```python
from build123d import *

# Parameters (mm, degrees)
SKETCH1_W           = 45.21
SKETCH1_H           = 20.09
SKETCH1_R           = 1.13
BOSS_EXTRUDE1_DEPTH = 1.2
SKETCH2_W           = 6
SKETCH2_H           = 16
BOSS_EXTRUDE3_DEPTH = 9
CUT_EXTRUDE1_REACH  = 32.67
SKETCH5_W           = 8
SKETCH5_H           = 9
BOSS_EXTRUDE5_DEPTH = 4


with BuildPart() as part:
    # Sketch1 → Boss-Extrude1 (new body)
    with BuildSketch(Plane(origin=(0, 0, 0), x_dir=(1, 0, 0), z_dir=(0, 1, 0))):
        Rectangle(SKETCH1_W, SKETCH1_H)
        with Locations(Location((11.835, 7.785, 0), (0, 0, 270))):
            Circle(SKETCH1_R, mode=Mode.SUBTRACT)
        with Locations(Location((-20.675, -7.635, 0), (0, 0, 270))):
            Circle(SKETCH1_R, mode=Mode.SUBTRACT)
    extrude(amount=BOSS_EXTRUDE1_DEPTH)

    # Sketch2 → Boss-Extrude3 (add)
    with BuildSketch(Plane(origin=(0, 1.2, 0), x_dir=(1, 0, 0), z_dir=(0, 1, 0))):
        with Locations((18.605, 0)):
            Rectangle(SKETCH2_W, SKETCH2_H)
    extrude(amount=BOSS_EXTRUDE3_DEPTH)

    # Sketch4 → Cut-Extrude1 (cut, up to next)
    with BuildSketch(Plane.XY.offset(8), mode=Mode.PRIVATE) as cut_extrude1_sk1:
        Polygon((15.605, 5.7), (16.788227765, 10.2), (15.605, 10.2), align=None)
    cut_extrude1_tool1 = extrude(cut_extrude1_sk1.sketch, amount=-CUT_EXTRUDE1_REACH, mode=Mode.PRIVATE) & part.part
    # Sketch4 → Cut-Extrude1 (cut, up to next)
    with BuildSketch(Plane.XY.offset(8), mode=Mode.PRIVATE) as cut_extrude1_sk2:
        Polygon((20.317369028, 10.2), (21.605, 5.7), (21.605, 10.2), align=None)
    cut_extrude1_tool2 = extrude(cut_extrude1_sk2.sketch, amount=-CUT_EXTRUDE1_REACH, mode=Mode.PRIVATE) & part.part
    add(cut_extrude1_tool1.solids().sort_by_distance((15.999409, 8.7, 8))[0], mode=Mode.SUBTRACT)
    add(cut_extrude1_tool2.solids().sort_by_distance((21.17579, 8.7, 8))[0], mode=Mode.SUBTRACT)

    # Sketch5 → Boss-Extrude5 (add)
    with BuildSketch(Plane(origin=(0, 1.2, 0), x_dir=(1, 0, 0), z_dir=(0, 1, 0))):
        with Locations((-13.605, -5.545)):
            Rectangle(SKETCH5_W, SKETCH5_H)
    extrude(amount=BOSS_EXTRUDE5_DEPTH)


solid = part.part
```
Verification items for the finished model (mm, model axes). A direction names the side the tool comes from. Round coordinates to 2 decimals unless told otherwise and drop trailing zeros. Order: outer loops, then holes, each group sorted by start corner. A loop starts at its lowest first (then second) coordinate and runs counter-clockwise, first axis right, second up. Notation, with made-up numbers: (25, 74.5) -> (77, 74.5) arc R12 ccw to (77, 80.5) -> close; hole circle Ø3 at (43, 12.25). An arc over 180 degrees is marked (long way). Put each result on its own line as item: value. Start each with the question number.
(1) Section check B-B (z = 5.5). Enter the section's corners in (x, y) (3 decimals).
(2) Material ranges on line 1 along X through (y, z) = (5, 5.75) (3 decimals); line 2 along Z through (x, y) = (-14, 5) (3 decimals); line 3 along Y through (x, z) = (13, 0.75), recorded low to high.
(3) Section check D-D (z = -5.25). Enter the section's corners in (x, y) (3 decimals), then the cut area to 3 significant figures.
(4) Section check A-A (y = 4). Enter the section's corners in (x, z) (3 decimals), then the cut area to 3 significant figures.
(5) Draft check along Z on faces 5 (the face through (-9.605, 3, 6)), 6 (the face through (-14, 3, 1.045)), 7 (the face through (19, 6, 8)), 8 (the face through (12.599, 0.592, -8.618)). Enter one of: +Z half, -Z half, draft (parallel to the pull), parting line (faces both ways), or undercut.
(6) Section check C-C (x = -15). Enter the section's corners in (y, z) (3 decimals), then the cut area to 3 significant figures.
(7) Tool access check on faces 1 (the face through (-17.605, 3, 6)), 2 (the face through (15.605, 3, 0)), 3 (the face through (19, 6, -8)), 4 (the face through (21.605, 3, 0)). Record the directions out of +Z, -Z, +X, -X, +Y, -Y that give a thin tool (end or side, any length) a straight path to the whole face; none if there is none.
(8) Depth check by flat-ended pin: pin 1 Ø1.2 at (x, y) = (-15, 3.5) entering from -Z (3 decimals); pin 2 Ø2 at (x, z) = (-20.675, 7.635) entering from -Y; pin 3 Ø5 at (y, z) = (4.5, 0) entering from +X (3 decimals); pin 4 Ø6 at (x, z) = (-10.5, 0) entering from +Y. Enter the tip coordinate at first touch or a pass-through.
Completed:
1. outline: (-22.605, 0) -> (22.605, 0) -> (22.605, 1.2) -> (21.605, 1.2) -> (21.605, 5.7) -> (20.317, 10.2) -> (16.788, 10.2) -> (15.605, 5.7) -> (15.605, 1.2) -> (-9.605, 1.2) -> (-9.605, 5.2) -> (-17.605, 5.2) -> (-17.605, 1.2) -> (-22.605, 1.2) -> close
2. line 1: x = -17.605 to -9.605, 15.605 to 21.605
2. line 2: z = 1.045 to 10.045
2. line 3: y = 0 to 1.2
3. outline: (-22.605, 0) -> (22.605, 0) -> (22.605, 1.2) -> (21.605, 1.2) -> (21.605, 5.7) -> (20.317, 10.2) -> (16.788, 10.2) -> (15.605, 5.7) -> (15.605, 1.2) -> (-22.605, 1.2) -> close
3. area: 103 mm2
4. outline: (-17.605, 1.045) -> (-9.605, 1.045) -> (-9.605, 10.045) -> (-17.605, 10.045) -> close; (15.605, -8) -> (21.605, -8) -> (21.605, 8) -> (15.605, 8) -> close
4. area: 168 mm2
5. face 5: draft
5. face 6: -Z half
5. face 7: +Z half
5. face 8: undercut
6. outline: (0, -10.045) -> (1.2, -10.045) -> (1.2, 1.045) -> (5.2, 1.045) -> (5.2, 10.045) -> (0, 10.045) -> close
6. area: 60.1 mm2
7. face 1: +Z, -Z, -X, +Y
7. face 2: +Z, -Z, +Y
7. face 3: -Z, +X, -X, +Y
7. face 4: +Z, -Z, +X, +Y
8. pin 1: stops at z = 1.045
8. pin 2: passes through
8. pin 3: stops at x = 21.605
8. pin 4: stops at y = 5.2
